CAD build for the part. Positions are in the model's coordinates, mm. Face numbers are marked on the shaded views. A direction names the side the tool comes from. Round coordinates to 2 decimals unless told otherwise and drop trailing zeros. Loops run counter-clockwise (first coordinate to the right, second up) from the corner with the lowest first, then second, coordinate; pieces in that order, holes last. Notation, with made-up numbers: M 30,26.25 L 47,26.25 A9 ccw 47,37.25 Z; hole C 29,51.25 d5. An arc over 180 degrees is marked long. Use one line per item in the form item = value.
from build123d import *

# Parameters (mm, degrees)
F0_W     = 4
F0_H     = 543
F1_DEPTH = 825
F2_W     = 6
F2_H     = 543
F3_DEPTH = 4


with BuildPart() as f1:
    # F0 (on Front) → F1 (new body)
    with BuildSketch(Plane.XZ):
        with Locations((2, 271.5)):
            Rectangle(F0_W, F0_H)
        Polygon((4, 0), (0, 0), (74.003571, -75.660426), (76.831998, -72.831998), align=None)
    extrude(amount=F1_DEPTH)

    # F2 (on face) → F3 (join)
    with BuildSketch(Plane.YZ.offset(4)):
        with Locations((3, 271.5)):
            Rectangle(F2_W, F2_H)
        with Locations((-828, 271.5)):
            Rectangle(F2_W, F2_H)
    extrude(amount=-F3_DEPTH)


solid = f1.part
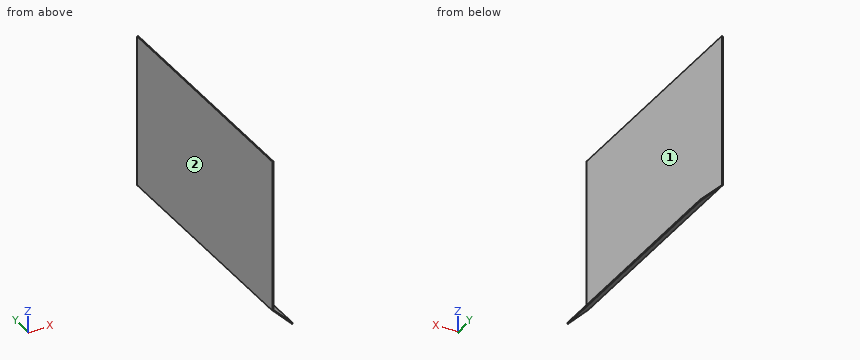
1. Drop flat-ended pins along their axis: P1, Ø22.5, axis at x = 50, z = -48.5, coming from the +Y side; P2, Ø1, axis at x = 26.5, y = -253.5, coming from the -Z side; P3, Ø6, axis at x = 48, y = -139, coming from the +Z side. Give the stop position or say it passes through.
Completed:
P1 = 0
P2 = -27.6
P3 = -41
2. Probe line 1 along X through (y, z) = (-487, 212); line 2 along Z through (x, y) = (24.5, -356.5); line 3 along Z through (x, y) = (16, -275.5). List the from-to ranges inside material, lowest first. Write a range as from..to.
Completed:
line_1 = 0..4
line_2 = -25.05..-20.5
line_3 = -16.36..-12
3. Cut at B-B on y = -191. Write the cut outline in (x, z), and give its area (3 significant figures).
Completed:
outline = M 0,0 L 74,-75.66 L 76.83,-72.83 L 4,0 L 4,543 L 0,543 Z
area = 2,530 mm2
4. Cut at A-A on z = 86. Write the cut outline in (x, y), and give its area (3 significant figures).
Completed:
outline = M 0,-831 L 4,-831 L 4,6 L 0,6 Z
area = 3,350 mm2
5. Cut at C-C on x = 21.5. Write the cut outline in (y, z), and give its area (3 significant figures).
Completed:
outline = M -825,-21.98 L 0,-21.98 L 0,-17.5 L -825,-17.5 Z
area = 3,700 mm2
6. Tool access for the marked faces 1 and 2: list every direction of +Z, -Z, +X, -X, +Y, -Y with a clear straight run to the whole face (end or side of a thin tool).
Completed:
face_1 = +Z, +X, +Y, -Y
face_2 = +Z, -Z, -X, +Y, -Y
